from build123d import *

# Parameters (mm, degrees)
SKETCH1_W           = 25
SKETCH1_H           = 25
SKETCH1_R           = 2.025
BOSS_EXTRUDE1_DEPTH = 2
SKETCH2_W           = 25
SKETCH2_H           = 2
BOSS_EXTRUDE2_DEPTH = 10.5
SKETCH3_W           = 25
SKETCH3_H           = 2
BOSS_EXTRUDE3_DEPTH = 55
FILLET1_R           = 3
FILLET2_R           = 2
FILLET3_R           = 1
BOSS_EXTRUDE4_DEPTH = 25
FILLET4_R           = 3
FILLET5_R           = 2
SKETCH6_R           = 5.5
CUT_EXTRUDE1_DEPTH  = 95.523989327
FILLET6_R           = 6


with BuildPart() as part:
    # Sketch1 → Boss-Extrude1 (new body)
    with BuildSketch(Plane.XY):
        Rectangle(SKETCH1_W, SKETCH1_H)
        with Locations((-7.5, 7.5)):
            Circle(SKETCH1_R, mode=Mode.SUBTRACT)
        with Locations((7.5, 7.5)):
            Circle(SKETCH1_R, mode=Mode.SUBTRACT)
        with Locations((7.5, -7.5)):
            Circle(SKETCH1_R, mode=Mode.SUBTRACT)
        with Locations((-7.5, -7.5)):
            Circle(SKETCH1_R, mode=Mode.SUBTRACT)
    extrude(amount=BOSS_EXTRUDE1_DEPTH)

    # Sketch2 → Boss-Extrude2 (add)
    with BuildSketch(Plane.XZ.offset(12.5)):
        with Locations((0, 1)):
            Rectangle(SKETCH2_W, SKETCH2_H)
    extrude(amount=BOSS_EXTRUDE2_DEPTH)

    # Sketch3 → Boss-Extrude3 (add)
    with BuildSketch(Plane.XY.offset(2)):
        with Locations((0, -22)):
            Rectangle(SKETCH3_W, SKETCH3_H)
    extrude(amount=BOSS_EXTRUDE3_DEPTH)

    # Fillet1
    fillet1_edges = [part.edges().sort_by_distance(p)[0] for p in [
        (-12.5, 12.5, 1),
        (12.5, 12.5, 1),
    ]]
    fillet(fillet1_edges, radius=FILLET1_R)

    # Fillet2
    fillet2_edges = [part.edges().sort_by_distance(p)[0] for p in [
        (0, -23, 0),
    ]]
    fillet(fillet2_edges, radius=FILLET2_R)

    # Fillet3
    fillet3_edges = [part.edges().sort_by_distance(p)[0] for p in [
        (0, -21, 2),
    ]]
    fillet(fillet3_edges, radius=FILLET3_R)

    # Sketch5 → Boss-Extrude4 (add)
    with BuildSketch(Plane.ZY.offset(12.5)):
        Polygon((57, -21), (86.708042062, -25.175193029), (86.42969586, -27.155729166), (57, -23.019655145), (56.721653798, -22.980536137), align=None)
    extrude(amount=-BOSS_EXTRUDE4_DEPTH)

    # Fillet4
    fillet4_edges = [part.edges().sort_by_distance(p)[0] for p in [
        (0, -21, 57),
    ]]
    fillet(fillet4_edges, radius=FILLET4_R)

    # Fillet5
    fillet5_edges = [part.edges().sort_by_distance(p)[0] for p in [
        (0, -23, 56.860146376),
    ]]
    fillet(fillet5_edges, radius=FILLET5_R)

    # Sketch6 → Cut-Extrude1 (cut, through all)
    with BuildSketch(Plane.XZ.offset(23)):
        with Locations(Location((0, 33, 0), (0, 0, 270))):
            Circle(SKETCH6_R)
    extrude(amount=-CUT_EXTRUDE1_DEPTH, mode=Mode.SUBTRACT)

    # Fillet6
    fillet6_edges = [part.edges().sort_by_distance(p)[0] for p in [
        (12.5, -26.165461098, 86.568868961),
        (-12.5, -26.165461098, 86.568868961),
    ]]
    fillet(fillet6_edges, radius=FILLET6_R)


solid = part.part
CAD build for the part. Positions are in the model's coordinates, mm. A direction names the side the tool comes from. Round coordinates to 2 decimals unless told otherwise and drop trailing zeros. Write each loop counter-clockwise with the first axis right and the second up, starting at its lowest first coordinate (ties: lowest second). Pieces come first, ordered by that corner, then holes. Notation, with made-up numbers: M 84.25,16 L 100.25,16 A21 cw 100.25,23 Z; hole C 85,7 d8. An arc over 180 degrees is marked long. Use a Markdown table: item, result. Add a question column.
1. Flat gauge pins, fed straight in: P1, Ø6, axis at x = 2, y = 8, coming from the +Z side; P2, Ø3, axis at x = -9.5, z = 46, coming from the -Y side; P3, Ø6.5, axis at x = 7.5, y = 7.5, coming from the -Z side; P4, Ø3, axis at x = -8.5, z = 73.5, coming from the +Y side. Where does each tip first touch, or does it go through?
2. Drill centre lines: probe 1 along Y at (x, z) = (7.5, 0.75) (3 decimals); probe 2 along Y at (x, z) = (7.5, 1.1) (3 decimals); probe 3 along Z at (x, y) = (8.5, -17). Where is each one in solid material? Low to high.
3. 3-axis set-ups, long thin cutter, end or side, ignore diameter. For faces 4 (the face through (-6, -23, 29)), 5 (the face through (-6, -21, 30)), 6 (the face through (12.5, -22, 29)): which of +Z, -Z, +X, -X, +Y, -Y reach the whole face in a straight line?
4. Slice it at A-A on x = 0. Give the cut face in (y, z).
5. Slice it at D-D on z = 44. Give the cut face in (x, y), then the cut area to 3 significant figures.
6. Slice it at B-B on y = 7.5. Give the cut face in (x, z) (3 decimals), then the cut area to 3 significant figures.
7. Pull direction Y, two halves, no side cores. Call faces 1 (the face through (-0.175, -23.073, 71.751)), 2 (the face through (-7.939, 5.523, 0.986)), 3 (the face through (10.7, -25.94, 84.87)): released by +Y, released by -Y, zero draft, split by the parting line, or undercut.
8. Slice it at C-C on x = 7.75. Give the cut face in (y, z).
Reply:
| question | item | result |
|---|---|---|
| 1 | P1 | stops at z = 2 |
| 1 | P2 | stops at y = -23 |
| 1 | P3 | stops at z = 0 |
| 1 | P4 | stops at y = -23.11 |
| 2 | probe 1 | y = -22.561 to -9.525, -5.475 to 5.475, 9.525 to 12.5 |
| 2 | probe 2 | y = -22.786 to -9.525, -5.475 to 5.475, 9.525 to 12.5 |
| 2 | probe 3 | z = 0 to 2 |
| 3 | face 4 | -Z, +X, -X, -Y |
| 3 | face 5 | +Z, +X, -X, +Y |
| 3 | face 6 | +Z, -Z, +X, +Y, -Y |
| 4 | outline | M -27.16,86.43 L -23.02,57 A2 cw -23,56.72 L -23,38.5 L -21,38.5 L -21,56.79 A3 ccw -21.03,57.21 L -25.18,86.71 Z; M -23,2 A2 ccw -21,0 L 12.5,0 L 12.5,2 L -20,2 A1 cw -21,3 L -21,27.5 L -23,27.5 Z |
| 5 | outline | M -12.5,-23 L 12.5,-23 L 12.5,-21 L -12.5,-21 Z |
| 5 | area | 50.0 mm^2 |
| 6 | outline | M -12.5,0 L -9.525,0 L -9.525,2 L -12.5,2 Z; M -5.475,0 L 5.475,0 L 5.475,2 L -5.475,2 Z; M 9.525,0 L 12.5,0 L 12.5,2 L 9.525,2 Z |
| 6 | area | 33.8 mm^2 |
| 7 | face 1 | released by +Y |
| 7 | face 2 | undercut |
| 7 | face 3 | released by -Y |
| 8 | outline | M -27.14,86.3 L -23.02,57 A2 cw -23,56.72 L -23,2 A2 ccw -21,0 L -9.51,0 L -9.51,2 L -20,2 A1 cw -21,3 L -21,56.79 A3 ccw -21.03,57.21 L -25.16,86.58 Z; M -5.49,0 L 5.49,0 L 5.49,2 L -5.49,2 Z; M 9.51,0 L 12.5,0 L 12.5,2 L 9.51,2 Z |
